from build123d import *

# Parameters (mm, degrees)
SKETCH_W        = 20
SKETCH_H        = 20
PAD_DEPTH       = 5
SKETCH001_W     = 5
SKETCH001_H     = 6
PAD001_DEPTH    = 10
SKETCH002_R     = 1.6
POCKET_DEPTH    = 12.501
SKETCH003_R     = 1.5
POCKET001_DEPTH = 5.001
FILLET_R        = 3
FILLET001_R     = 2


with BuildPart() as part:
    # Sketch → Pad (new body)
    with BuildSketch(Plane.XY):
        with Locations((-10, 10)):
            Rectangle(SKETCH_W, SKETCH_H)
    extrude(amount=PAD_DEPTH)

    # Sketch001 (on Face6 of Pad) → Pad001 (join)
    with BuildSketch(Plane.XY.offset(5)):
        with Locations((-10, 10)):
            Rectangle(SKETCH001_W, SKETCH001_H)
    extrude(amount=PAD001_DEPTH)

    # Sketch002 (on Face8 of Pad001) → Pocket (cut, through all)
    with BuildSketch(Plane.YZ.offset(-7.5)):
        with Locations((10, 12.205362)):
            Circle(SKETCH002_R)
    extrude(amount=-POCKET_DEPTH, mode=Mode.SUBTRACT)

    # Sketch003 (on Face5 of Pocket) → Pocket001 (cut, through all)
    with BuildSketch(Plane.XY.offset(5)):
        with Locations((-10, 15.417424)):
            Circle(SKETCH003_R)
        with Locations((-10, 4.582576)):
            Circle(SKETCH003_R)
    extrude(amount=-POCKET001_DEPTH, mode=Mode.SUBTRACT)

    # Fillet
    fillet_edges = [part.edges().sort_by_distance(p)[0] for p in [
        (0, 10, 5),
        (-10, 0, 5),
        (-20, 10, 5),
        (-10, 20, 5),
    ]]
    fillet(fillet_edges, radius=FILLET_R)

    # Fillet001
    fillet001_edges = [part.edges().sort_by_distance(p)[0] for p in [
        (-10, 7, 15),
        (-10, 13, 15),
    ]]
    fillet(fillet001_edges, radius=FILLET001_R)


solid = part.part
Geometry check sheet. Reference: the model listing, model coordinates, mm. A direction names the side the tool comes from. Give positions to 0.01 mm unless a question says otherwise; leave off trailing zeros. Loops run counter-clockwise (first coordinate to the right, second up) from the corner with the lowest first, then second, coordinate; pieces in that order, holes last. Notation, with made-up numbers: (-3.5, 79) -> (34.5, 79) arc R23 ccw to (34.5, 113) -> close; hole circle Ø5 at (-30.5, -35.5). An arc over 180 degrees is marked (long way). Answer in a Markdown table with one row per item. Add a question column.
1) Cross-section at B-B on x = -9.25. Record the boundary of the cut face in (y, z), and give its area (3 significant figures).
2) Draft check along Y on faces 1 (the face through (-10, 10, 0)), 2 (the face through (-9.86, 0.86, 4.1)), 3 (the face through (-10.325, 13.953, 2.535)), 4 (the face through (-9.86, 19.14, 4.1)). Enter one of: pulls with the +Y half, pulls with the -Y half, needs draft (parallel to the pull), parting line crosses it, or undercut.
3) Cross-section at D-D on z = 4. Record the boundary of the cut face in (x, y), and give its area (3 significant figures).
4) Set-up check for faces 5 (the face through (0, 10, 1)), 6 (the face through (-10, 7, 9)), 7 (the face through (-7.5, 10, 10)), 8 (the face through (-10, 13, 9)), 9 (the face through (-12.5, 10, 10)): record each of +Z, -Z, +X, -X, +Y, -Y from which the full face is reachable in a straight line by a thin tool's end or side.
5) Material ranges on probe 1 along Y at (x, z) = (-10, 2.4); probe 2 along Z at (x, y) = (-8.7, 10); probe 3 along X at (y, z) = (8.75, 10.75), recorded low to high. Write a range as from..to.
6) Gauge pin test, flat ends, axial feed: P1, Ø2.5, axis at x = -10, y = 4.58, coming from the -Z side; P2, Ø10, axis at x = -13.5, y = 11.5, coming from the +Z side; P3, Ø4, axis at y = 10, z = 12.21, coming from the -X side; P4, Ø3, axis at x = -11.5, z = 6, coming from the -Y side. Record the tip position at first contact, or that the pin passes through.
7) Cross-section at A-A on y = 10. Record the boundary of the cut face in (x, z).
8) Cross-section at C-C on x = -13.5. Record the boundary of the cut face in (y, z), and give its area (3 significant figures).
Outcome:
| question | item | result |
|---|---|---|
| 1 | outline | (0, 0) -> (3.28, 0) -> (3.28, 5) -> (3, 5) arc R3 ccw to (0, 2) -> close; (5.88, 0) -> (14.12, 0) -> (14.12, 5) -> (13, 5) -> (13, 13) arc R2 ccw to (11, 15) -> (9, 15) arc R2 ccw to (7, 13) -> (7, 5) -> (5.88, 5) -> close; (16.72, 0) -> (20, 0) -> (20, 2) arc R3 ccw to (17, 5) -> (16.72, 5) -> close; hole circle Ø3.2 at (10, 12.21) |
| 1 | area | 120 mm^2 |
| 2 | face 1 | needs draft |
| 2 | face 2 | pulls with the -Y half |
| 2 | face 3 | undercut |
| 2 | face 4 | pulls with the +Y half |
| 3 | outline | (-19.24, 0.76) -> (-0.76, 0.76) -> (-0.76, 19.24) -> (-19.24, 19.24) -> close; hole circle Ø3 at (-10, 4.58); hole circle Ø3 at (-10, 15.42) |
| 3 | area | 327 mm^2 |
| 4 | face 5 | +Z, -Z, +X, +Y, -Y |
| 4 | face 6 | +Z, +X, -X, -Y |
| 4 | face 7 | +Z, +X, +Y, -Y |
| 4 | face 8 | +Z, +X, -X, +Y |
| 4 | face 9 | +Z, -X, +Y, -Y |
| 5 | probe 1 | y = 0.03..3.08, 6.08..13.92, 16.92..19.97 |
| 5 | probe 2 | z = 0..10.61, 13.81..15 |
| 5 | probe 3 | x = -12.5..-7.5 |
| 6 | P1 | passes through |
| 6 | P2 | stops at z = 15 |
| 6 | P3 | stops at x = -12.5 |
| 6 | P4 | stops at y = 1.34 |
| 7 | outline | (-20, 0) -> (0, 0) -> (0, 2) arc R3 ccw to (-3, 5) -> (-7.5, 5) -> (-7.5, 10.61) -> (-12.5, 10.61) -> (-12.5, 5) -> (-17, 5) arc R3 ccw to (-20, 2) -> close; (-12.5, 13.81) -> (-7.5, 13.81) -> (-7.5, 15) -> (-12.5, 15) -> close |
| 8 | outline | (0, 0) -> (20, 0) -> (20, 2) arc R3 ccw to (17, 5) -> (3, 5) arc R3 ccw to (0, 2) -> close |
| 8 | area | 96.1 mm^2 |
